```python
from build123d import *

# Parameters (mm, degrees)
BOSS_EXTRUDE1_DEPTH                                 = 15
M4_CLEARANCE_HOLE1_D                                = 4.5
M4_CLEARANCE_HOLE1_DEPTH                            = 16
M4_CLEARANCE_HOLE1_TIP                              = 1.351936393
CBORE_FOR_M3_HEX_SOCKET_HEAD_CAP_SCREW1_D           = 3.4
CBORE_FOR_M3_HEX_SOCKET_HEAD_CAP_SCREW1_CBORE_D     = 6.5
CBORE_FOR_M3_HEX_SOCKET_HEAD_CAP_SCREW1_CBORE_DEPTH = 6
FILLET1_R                                           = 5
CHAMFER1_SIZE                                       = 1
SKETCH6_R                                           = 5
CUT_EXTRUDE1_DEPTH                                  = 5
SKETCH7_R                                           = 5
CUT_EXTRUDE2_DEPTH                                  = 4
BOSS_EXTRUDE2_START                                 = -0.4
SKETCH8_R                                           = 2.25
BOSS_EXTRUDE2_DEPTH                                 = 0.4


with BuildPart() as part:
    # Sketch1 → Boss-Extrude1 (new, symmetric)
    with BuildSketch(Plane(origin=(0, 0, 0), x_dir=(0, 0, -1), z_dir=(1, 0, 0))):
        Polygon((8, -19), (8, -30), (0, -30), (0, 30), (8, 30), (8, 19), (8.5, 19), (8.5, 11), (8, 11), (8, -11), (8.5, -11), (8.5, -19), align=None)
    extrude(amount=BOSS_EXTRUDE1_DEPTH, both=True)

    # M4 Clearance Hole1
    with Locations(Plane.XY):
        with Locations((0, -15), (0, 15)):
            Hole(M4_CLEARANCE_HOLE1_D / 2, depth=M4_CLEARANCE_HOLE1_DEPTH)
            with Locations((0, 0, -(M4_CLEARANCE_HOLE1_DEPTH + M4_CLEARANCE_HOLE1_TIP / 2))):  # 118° drill point
                Cone(0, M4_CLEARANCE_HOLE1_D / 2, M4_CLEARANCE_HOLE1_TIP, mode=Mode.SUBTRACT)

    # CBORE for M3 Hex Socket Head Cap Screw1 (through all)
    with Locations(Plane(origin=(0, 0, -8.5), x_dir=(-1, 0, 0), z_dir=(0, 0, -1))):
        with Locations((0, 0)):
            CounterBoreHole(CBORE_FOR_M3_HEX_SOCKET_HEAD_CAP_SCREW1_D / 2, CBORE_FOR_M3_HEX_SOCKET_HEAD_CAP_SCREW1_CBORE_D / 2, CBORE_FOR_M3_HEX_SOCKET_HEAD_CAP_SCREW1_CBORE_DEPTH)

    # Fillet1
    fillet1_edges = [part.edges().sort_by_distance(p)[0] for p in [
        (-15, -30, -4),
        (-15, 30, -4),
        (15, 30, -4),
        (15, -30, -4),
    ]]
    fillet(fillet1_edges, radius=FILLET1_R)

    # Chamfer1
    chamfer1_edges = [part.edges().sort_by_distance(p)[0] for p in [
        (0, 30, 0),
        (-15, 0, 0),
        (0, -30, 0),
        (15, 0, 0),
        (-13.535533906, -28.535533906, 0),
        (13.535533906, -28.535533906, 0),
        (13.535533906, 28.535533906, 0),
        (-13.535533906, 28.535533906, 0),
    ]]
    chamfer(chamfer1_edges, length=CHAMFER1_SIZE)

    # Sketch6 → Cut-Extrude1 (cut)
    with BuildSketch(Plane.XY):
        with Locations((8, -23)):
            Circle(SKETCH6_R)
    extrude(amount=-CUT_EXTRUDE1_DEPTH, mode=Mode.SUBTRACT)

    # Sketch7 → Cut-Extrude2 (cut)
    with BuildSketch(Plane.XY):
        with Locations((0, 15)):
            Circle(SKETCH7_R)
        with Locations((0, -15)):
            Circle(SKETCH7_R)
    extrude(amount=-CUT_EXTRUDE2_DEPTH, mode=Mode.SUBTRACT)

    # Sketch8 → Boss-Extrude2 (add)
    with BuildSketch(Plane.XY.offset(-4).offset(BOSS_EXTRUDE2_START)):
        with Locations((0, 15)):
            Circle(SKETCH8_R)
        with Locations((0, -15)):
            Circle(SKETCH8_R)
    extrude(amount=BOSS_EXTRUDE2_DEPTH)


solid = part.part
```
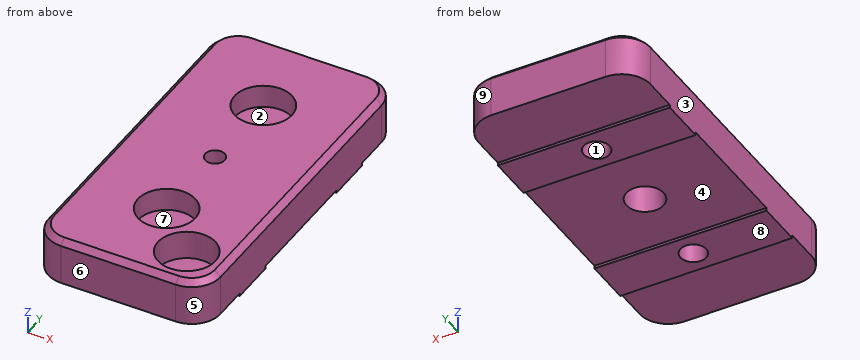
CAD build for the part. Positions are in the model's coordinates, mm. Face numbers are marked on the shaded views. A direction names the side the tool comes from. Round coordinates to 2 decimals unless told otherwise and drop trailing zeros. Order: outer loops, then holes, each group sorted by start corner. A loop starts at its lowest first (then second) coordinate and runs counter-clockwise, first axis right, second up. Notation, with made-up numbers: (3, 64) -> (48, 64) arc R24 cw to (48, 78) -> close; hole circle Ø6 at (-24, 79). An arc over 180 degrees is marked (long way). One line per question, with ' | ' between items.
Q1. Drop flat-ended pins along their axis: pin 1 (12 mm diameter, centred on x = -6.5, y = -26.5, fed in from -Z); pin 2 (2.5 mm diameter, centred on x = 0, y = 15, fed in from +Z); pin 3 (3 mm diameter, centred on x = 1, y = -1, fed in from +Z); pin 4 (3 mm diameter, centred on x = 0, y = -0.5, fed in from -Z). Give the stop position or say it passes through.
Completed:
pin 1: stops at z = -8 | pin 2: stops at z = -4 | pin 3: stops at z = 0 | pin 4: stops at z = -2.5
Q2. Which spindle directions (+Z, -Z, +X, -X, +Y, -Y) get a long thin tool onto all of the face, cutting with end or side? Do the marked faces 1, 2, 3, 4 and 5. Say none if no direction does.
Completed:
face 1: -Z | face 2: +Z | face 3: +Z, -Z, -X, +Y, -Y | face 4: -Z, +X, -X | face 5: +Z, -Z, +X, -Y
Q3. Slice it at D-D (x = -7.25). Write the cut outline in (y, z), then the cut area to 3 significant figures.
Completed:
outline: (-30, -8) -> (-19, -8) -> (-19, -8.5) -> (-11, -8.5) -> (-11, -8) -> (11, -8) -> (11, -8.5) -> (19, -8.5) -> (19, -8) -> (30, -8) -> (30, -1) -> (29, 0) -> (-29, 0) -> (-30, -1) -> close | area: 487 mm^2
Q4. Slice it at B-B (y = -23). Write the cut outline in (x, z), then the cut area to 3 significant figures.
Completed:
outline: (-15, -8) -> (15, -8) -> (15, -1) -> (14, 0) -> (13, 0) -> (13, -5) -> (3, -5) -> (3, 0) -> (-14, 0) -> (-15, -1) -> close | area: 189 mm^2
Q5. Two-plate mould, pull along Y, no slides. Class the marked faces 6, 7, 8 and 9: released by +Y, released by -Y, zero draft, split by the parting line, or undercut.
Completed:
face 6: released by -Y | face 7: undercut | face 8: zero draft | face 9: released by +Y
Q6. Probe probe 1 along Y at (x, z) = (0, -5.4); probe 2 along Y at (x, z) = (0, -1.45); probe 3 along Z at (x, y) = (-4, -1.5). List the from-to ranges inside material, lowest first.
Completed:
probe 1: y = -30 to -17.25, -12.75 to -3.25, 3.25 to 12.75, 17.25 to 30 | probe 2: y = -30 to -20, -10 to -1.7, 1.7 to 10, 20 to 30 | probe 3: z = -8 to 0
Q7. Slice it at A-A (z = -1.75). Write the cut outline in (x, y).
Completed:
outline: (-15, -25) arc R5 ccw to (-10, -30) -> (10, -30) arc R5 ccw to (15, -25) -> (15, 25) arc R5 ccw to (10, 30) -> (-10, 30) arc R5 ccw to (-15, 25) -> close; hole circle Ø10 at (0, -15); hole circle Ø10 at (0, 15); hole circle Ø3.4 at (0, 0); hole circle Ø10 at (8, -23)
Q8. Slice it at C-C (y = 0). Write the cut outline in (x, z).
Completed:
outline: (-15, -8) -> (-3.25, -8) -> (-3.25, -2.5) -> (-1.7, -2.5) -> (-1.7, 0) -> (-14, 0) -> (-15, -1) -> close; (1.7, -2.5) -> (3.25, -2.5) -> (3.25, -8) -> (15, -8) -> (15, -1) -> (14, 0) -> (1.7, 0) -> close
